Autodesk Inventor part; units mm, degrees
ref_plane "YZ Plane" through (0, 0, 0) normal (1, 0, 0) x (0, 1, 0)
ref_plane "XZ Plane" through (0, 0, 0) normal (0, 1, 0) x (-1, 0, 0)
ref_plane "XY Plane" through (0, 0, 0) normal (0, 0, 1) x (1, 0, 0)
sketch "Sketch1" plane through (0, 0, 0) normal (0, 0, 1) x (1, 0, 0)
  line L0 (0, 0) -> (177.8, 0)
  line L1 (177.8, 0) -> (177.8, 101.6)
  line L2 (177.8, 101.6) -> (0, 101.6)
  line L3 (0, 101.6) -> (0, 0)
  arc A0 (25.4, 101.6) -> (0, 76.2) centre (25.4, 76.2) ccw
  arc A1 (177.8, 76.2) -> (152.4, 101.6) centre (152.4, 76.2) ccw
  arc A2 (152.4, 0) -> (177.8, 25.4) centre (152.4, 25.4) ccw
  arc A3 (0, 25.4) -> (25.4, 0) centre (25.4, 25.4) ccw
  circle A4 centre (88.9, 50.8) radius 6.35
  arc A5 (88.9, 85.09) -> (54.61, 50.8) centre (88.9, 50.8) ccw construction
  arc A6 (88.9, 88.9) -> (50.8, 50.8) centre (88.9, 50.8) ccw
  arc A7 (88.9, 81.28) -> (58.42, 50.8) centre (88.9, 50.8) ccw
  arc A8 (88.9, 81.28) -> (88.9, 88.9) centre (88.9, 85.09) ccw
  arc A9 (50.8, 50.8) -> (58.42, 50.8) centre (54.61, 50.8) ccw
  line L4 (88.9, 50.8) -> (54.61, 50.8) construction
  line L5 (88.9, 50.8) -> (88.9, 85.09) construction
  arc A10 (88.9, 20.32) -> (119.38, 50.8) centre (88.9, 50.8) ccw
  line L6 (88.9, 50.8) -> (123.19, 50.8) construction
  arc A11 (88.9, 16.51) -> (123.19, 50.8) centre (88.9, 50.8) ccw construction
  arc A12 (127, 50.8) -> (119.38, 50.8) centre (123.19, 50.8) ccw
  arc A13 (88.9, 12.7) -> (127, 50.8) centre (88.9, 50.8) ccw
  arc A14 (88.9, 20.32) -> (88.9, 12.7) centre (88.9, 16.51) ccw
  point P0 (0, 0)
  dimension "d2" = 177.8
  dimension "d3" = 101.6
  dimension "d4" = 50.8
  dimension "d5" = 50.8
  dimension "d6" = 50.8
  dimension "d7" = 50.8
  dimension "d8" = 12.7
  dimension "d9" = 50.8
  dimension "d10" = 88.9
  dimension "d11" = 34.29
  dimension "d12" = 90
  dimension "d13" = 7.62
  dimension "d14" = 360
  dimension "d15" = 0
  dimension "d16" = 0
extrude "Extrusion1" add sketch "Sketch1" along normal blind 3.175 contours A3 L3 A0 L2 A1 L1 A2 L0
properties part number "Front_plate"
CAD build for the part. Positions are in the model's coordinates, mm. A direction names the side the tool comes from. Round coordinates to 2 decimals unless told otherwise and drop trailing zeros. Write each loop counter-clockwise with the first axis right and the second up, starting at its lowest first coordinate (ties: lowest second). Pieces come first, ordered by that corner, then holes. Notation, with made-up numbers: (69.25, 30) -> (89.25, 30) arc R20 cw to (89.25, 45) -> close; hole circle Ø1 at (53, -3.5). An arc over 180 degrees is marked (long way). Answer in a Markdown table with one row per item. Add a question column.
Item 1: Saw through at A-A, the plane z = 1.2. Write the cut outline in (x, y), then the cut area to 3 significant figures.
Item 2: Which spindle directions (+Z, -Z, +X, -X, +Y, -Y) get a long thin tool onto all of the face, cutting with end or side? Do faces 1 (the face through (7.24, 93.96, 1.57)), 2 (the face through (116.14, 24.16, 1.57)). Say none if no direction does.
Item 3: Mould opens along X. For faces 3 (the face through (54.69, 46.99, 1.57)), 4 (the face through (88, 40, 3.175)), 5 (the face through (123.11, 54.61, 1.57)), 6 (the face through (170.56, 7.64, 1.57)) say: pulls with the +X half, pulls with the -X half, needs draft (parallel to the pull), parting line crosses it, or undercut.
Item 4: Saw through at B-B, the plane y = 16.51. Write the cut outline in (x, z) (3 decimals), then the cut area to 3 significant figures.
Item 5: Drill centre lines: line 1 (Y direction, x = 88.9, z = 1.55); line 2 (X direction, y = 45.5, z = 2.5); line 3 (Y direction, x = 74.5, z = 2.7). Where is each one in solid material? Low to high. Write a range as from..to.
Item 6: Drop a flat-ended pin along its axis: pin 1 Ø14.5 at (x, y) = (88.9, 50.8) entering from -Z. Give the stop position or say it passes through.
Item 7: Saw through at C-C, the plane x = 54.61. Write the cut outline in (y, z) (3 decimals).
Findings below:
| question | item | result |
|---|---|---|
| 1 | outline | (0, 25.4) arc R25.4 ccw to (25.4, 0) -> (152.4, 0) arc R25.4 ccw to (177.8, 25.4) -> (177.8, 76.2) arc R25.4 ccw to (152.4, 101.6) -> (25.4, 101.6) arc R25.4 ccw to (0, 76.2) -> close; hole (50.8, 50.8) arc R3.81 ccw to (58.42, 50.8) arc R30.48 cw to (88.9, 81.28) arc R3.81 ccw to (88.9, 88.9) arc R38.1 ccw to start; hole circle Ø12.7 at (88.9, 50.8); hole (88.9, 12.7) arc R38.1 ccw to (127, 50.8) arc R3.81 ccw to (119.38, 50.8) arc R30.48 cw to (88.9, 20.32) arc R3.81 ccw to start |
| 1 | area | 16,500 mm^2 |
| 2 | face 1 | +Z, -Z, -X, +Y |
| 2 | face 2 | +Z, -Z |
| 3 | face 3 | undercut |
| 3 | face 4 | needs draft |
| 3 | face 5 | undercut |
| 3 | face 6 | pulls with the +X half |
| 4 | outline | (1.607, 0) -> (85.09, 0) -> (85.09, 3.175) -> (1.607, 3.175) -> close; (105.507, 0) -> (176.193, 0) -> (176.193, 3.175) -> (105.507, 3.175) -> close |
| 4 | area | 489 mm^2 |
| 5 | line 1 | y = 0..12.7, 20.32..44.45, 57.15..81.28, 88.9..101.6 |
| 5 | line 2 | x = 0..85.4, 92.4..118.92, 126.63..177.8 |
| 5 | line 3 | y = 0..77.66, 86.07..101.6 |
| 6 | pin 1 | stops at z = 0 |
| 7 | outline | (0, 0) -> (46.99, 0) -> (46.99, 3.175) -> (0, 3.175) -> close; (67.407, 0) -> (101.6, 0) -> (101.6, 3.175) -> (67.407, 3.175) -> close |
